```python
from build123d import *

# Parameters (mm, degrees)
F1_DEPTH = 717.55


with BuildPart() as f1:
    # F0 (on Right) → F1 (new body)
    with BuildSketch(Plane.YZ):
        with BuildLine():
            Line((15.875, 5.514235), (15.875, -0.073765))
            Line((15.875, -0.073765), (44.45, -0.073765))
            Line((44.45, -0.073765), (44.45, 12.626235))
            Line((44.45, 12.626235), (38.1, 12.626235))
            Line((38.1, 12.626235), (2.237371, 8.32272))
            ThreePointArc((2.237371, 8.32272), (0.639964, 7.486476), (0, 5.800812))
            Line((0, 5.800812), (0, 5.514235))
            Line((0, 5.514235), (15.875, 5.514235))
        make_face()
    extrude(amount=F1_DEPTH)


solid = f1.part
```
Can you work these out from the model? Positions are in its coordinate system, mm. A direction names the side the tool comes from. Round coordinates to 2 decimals unless told otherwise and drop trailing zeros. Loops run counter-clockwise (first coordinate to the right, second up) from the corner with the lowest first, then second, coordinate; pieces in that order, holes last. Notation, with made-up numbers: (66.5, 86) -> (103.5, 86) arc R28 ccw to (103.5, 123) -> close; hole circle Ø2 at (60, 5.25). An arc over 180 degrees is marked (long way). One line per item, written item: value. Start each with the question number.
1. If we section it at A-A, the plane x = 377.5: Write out the boundary of the cut face in (y, z) (3 decimals), then the cut area to 3 significant figures.
2. If I drill on probe 1 along Y at (x, z) = (679.5, 5) (3 decimals); probe 2 along Z at (x, y) = (580.5, 2); probe 3 along Z at (x, y) = (224.5, 38), over which ranges is the centre line in solid material (lowest first)?
3. For faces 1 (the flat face through (354, 44.45, 6)), 2 (the flat face through (354, 8, 5.514)), which set-ups out of +Z, -Z, +X, -X, +Y, -Y let a thin tool reach every point of the face, with its end or its side?
4. If we section it at B-B, the plane z = 2: Write out the boundary of the cut face in (x, y) (3 decimals), then the cut area to 3 significant figures.
5. For pin 1 (2 mm diameter, centred on y = 13, z = 5.5, fed in from -X); pin 2 (3 mm diameter, centred on x = 132, y = 25, fed in from +Z); pin 3 (12.5 mm diameter, centred on x = 292.5, y = 6, fed in from -Z); pin 4 (6 mm diameter, centred on x = 338, z = 2, fed in from -Y) (3 decimals), each with a flat end and sliding along its axis, tell me the tip position at first contact or that it passes through.
Calculated:
1. outline: (0, 5.514) -> (15.875, 5.514) -> (15.875, -0.074) -> (44.45, -0.074) -> (44.45, 12.626) -> (38.1, 12.626) -> (2.237, 8.323) arc R2.54 ccw to (0, 5.801) -> close
1. area: 388 mm²
2. probe 1: y = 15.875 to 44.45
2. probe 2: z = 5.51 to 8.28
2. probe 3: z = -0.07 to 12.61
3. face 1: +Z, -Z, +X, -X, +Y
3. face 2: -Z, +X, -X, -Y
4. outline: (0, 15.875) -> (717.55, 15.875) -> (717.55, 44.45) -> (0, 44.45) -> close
4. area: 20,500 mm²
5. pin 1: stops at x = 0
5. pin 2: stops at z = 11.23
5. pin 3: stops at z = 5.51
5. pin 4: stops at y = 15.875
